from build123d import *

# Parameters (mm, degrees)
F0_R     = 4.7625
F1_DEPTH = 19.05
F4_R     = 2.413
F5_DEPTH = 19.051
F8_R     = 2.54
F9_DEPTH = 0.6096


# Not quite as in the source:
# - a fillet or chamfer that OpenCascade refuses, or shapes differently, is made with other operations: its cross-section is extruded or revolved along the edge and cut away or added


with BuildPart() as f1:
    # F0 (on Front) → F1 (new body)
    with BuildSketch(Plane.XZ):
        Circle(F0_R)
    extrude(amount=F1_DEPTH)

    # F4 (on face) → F5 (cut, through all)
    with BuildSketch(Plane.XZ):
        Circle(F4_R)
    extrude(amount=F5_DEPTH, mode=Mode.SUBTRACT)

    # F6: fillet of radius 4.7498 on 2 edges, made by hand

    # F6_s1 → F6_t2 (revolve, cut)
    with BuildSketch(Plane.XY):
        with BuildLine():
            ThreePointArc((4.7625, -4.0986778295), (4.1334732879, -1.7365119695), (2.413, 0))
            Line((2.413, 0), (4.7625, 0))
            Line((4.7625, 0), (4.7625, -4.0986778295))
        make_face()
    revolve(axis=Axis((0, 0, 0), (0, -1, 0)), mode=Mode.SUBTRACT)

    # F6_s3 → F6_t4 (revolve, cut)
    with BuildSketch(Plane.XY):
        with BuildLine():
            ThreePointArc((4.7625, -14.9513221705), (4.1334732879, -17.3134880305), (2.413, -19.05))
            Line((2.413, -19.05), (4.7625, -19.05))
            Line((4.7625, -19.05), (4.7625, -14.9513221705))
        make_face()
    revolve(axis=Axis((0, -19.05, 0), (0, -1, 0)), mode=Mode.SUBTRACT)

    # F8 (on offset) → F9 (cut)
    with BuildSketch(Plane.XZ.offset(14.9606)):
        Circle(F8_R)
    extrude(amount=-F9_DEPTH, mode=Mode.SUBTRACT)


solid = f1.part
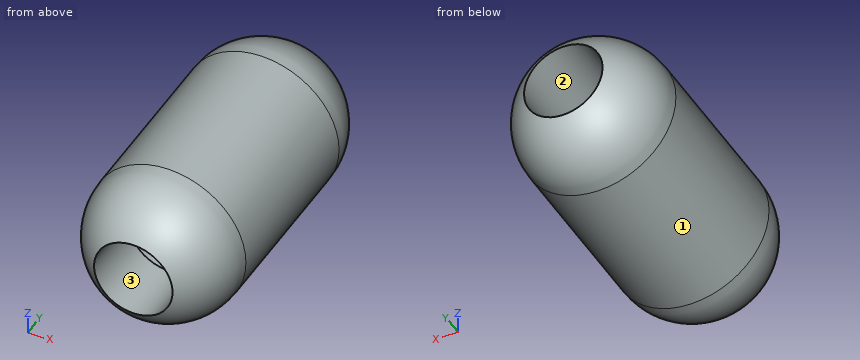
Could you check a few things on this model? Use its own coordinates, in mm. Face numbers are marked on the shaded views. Coordinates: 2 decimals unless noted, no trailing zeros. Write each loop counter-clockwise with the first axis right and the second up, starting at its lowest first coordinate (ties: lowest second). Pieces come first, ordered by that corner, then holes. Notation, with made-up numbers: M -3,-15 L 16,-15 A15 cw 16,-5 Z; hole C 86,75 d8. An arc over 180 degrees is marked long. One line per question, with ' | ' between items.
1) For pin 1 Ø5 at (x, y) = (-1.5, -16.5) entering from +Z; pin 2 Ø1 at (y, z) = (-2.5, 3) entering from -X, each with a flat end and sliding along its axis, tell me the tip position at first contact or that it passes through.
Checks:
pin 1: z = 4.76 | pin 2: x = -3.78
2) Imagine slicing it at A-A, the plane y = -14.75. Write out the boundary of the cut face in (x, z) (1 decimal).
Checks:
outline: C 0,0 d9.5; hole C 0,0 d5.1
3) I need wall thicknesses on probe 1 along Z at (x, y) = (0, -14.7); probe 2 along Z at (x, y) = (-1, -12); probe 3 along X at (y, z) = (-11.5, -1.5). Which ranges of each line are inside material? Lowest first, please. Write a range as [from, to].
Checks:
probe 1: [-4.76, -2.54], [2.54, 4.76] | probe 2: [-4.66, -2.2], [2.2, 4.66] | probe 3: [-4.52, -1.89], [1.89, 4.52]
4) If we mould it in two halves opening along Z, with no side actions, what happens to the marked faces 1, 2 and 3? For each: released by +Z, released by -Z, zero draft, split by the parting line, or undercut.
Checks:
face 1: split by the parting line | face 2: undercut | face 3: undercut
